Check sheet for the modelled part. Datum: model origin and axes. Units: mm. Give positions to 0.01 mm unless a question says otherwise; leave off trailing zeros. Order: outer loops, then holes, each group sorted by start corner. A loop starts at its lowest first (then second) coordinate and runs counter-clockwise, first axis right, second up. Notation, with made-up numbers: (34.5, 56.5) -> (55.5, 56.5) arc R13 ccw to (55.5, 78.5) -> close; hole circle Ø6 at (71.25, 31.25). An arc over 180 degrees is marked (long way). Answer in a Markdown table with one row per item. Add a question column.
(1) Go/stop test with flat-tipped pins: pin 1 (1.5 mm diameter, centred on x = 2, y = 5.5, fed in from -Z); pin 2 (1.5 mm diameter, centred on x = -5.5, y = 9, fed in from -Z); pin 3 (5.5 mm diameter, centred on x = 1.5, y = 5.5, fed in from -Z). Record where each tip stops, or that it passes through.
(2) Cross-section at A-A (x = -4). Record the cut outline in (y, z) (3 decimals), then the cut area to 3 significant figures.
(3) Thickness scan on L1, parallel to X at y = 8.75, z = -0.5; L2, parallel to Y at x = 4.5, z = 0.5; L3, parallel to Z at x = 1.25, y = 4.5. Record the ranges inside material, lowest first. Write a range as [from, to].
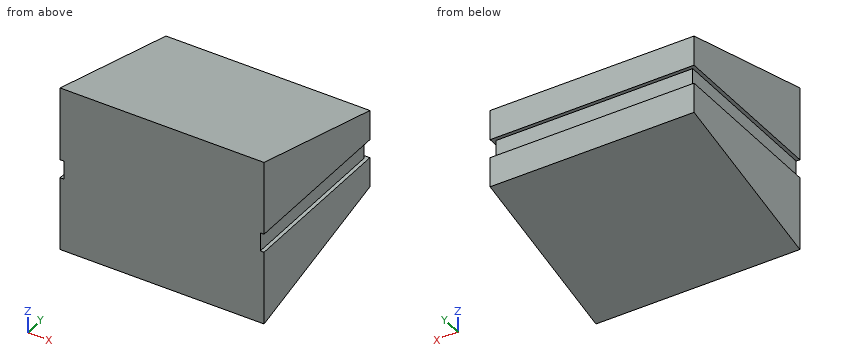
```python
from build123d import *

# Parameters (mm, degrees)
SKETCH4_W          = 13.8
SKETCH4_H          = 1.25
CUT_EXTRUDE1_DEPTH = 0.25
SKETCH5_W          = 1.25
SKETCH5_H          = 10.95
CUT_EXTRUDE2_DEPTH = 0.25
SKETCH6_W          = 1.25
SKETCH6_H          = 10.95
CUT_EXTRUDE3_DEPTH = 0.25


with BuildPart() as part:
    # Sketch1 → Loft1 section 0
    with BuildSketch(Plane(origin=(0, 0, 0), x_dir=(1, 0, 0), z_dir=(0, 1, 0))):
        with BuildLine():
            Line((-6.9, -5.61), (6.9, -5.61))
            Line((6.9, -5.61), (6.9, 5.61))
            Line((6.9, 5.61), (-6.9, 5.61))
            Line((-6.9, 5.61), (-6.9, -5.61))
        make_face()
    # Sketch2 → Loft1 section 1
    with BuildSketch(Plane(origin=(0, 11.2, 0), x_dir=(1, 0, 0), z_dir=(0, 1, 0))):
        with BuildLine():
            Line((-6.9, -2.651033308), (6.9, -2.651033308))
            Line((6.9, -2.651033308), (6.9, 2.648966692))
            Line((6.9, 2.648966692), (-6.9, 2.648966692))
            Line((-6.9, 2.648966692), (-6.9, -2.651033308))
        make_face()
    loft()

    # Sketch4 → Cut-Extrude1 (cut)
    with BuildSketch(Plane(origin=(0, 11.2, 0), x_dir=(1, 0, 0), z_dir=(0, 1, 0))):
        Rectangle(SKETCH4_W, SKETCH4_H)
    extrude(amount=-CUT_EXTRUDE1_DEPTH, mode=Mode.SUBTRACT)

    # Sketch5 → Cut-Extrude2 (cut)
    with BuildSketch(Plane(origin=(6.9, 0, 0), x_dir=(0, 0, -1), z_dir=(1, 0, 0))):
        with Locations((0, 5.475)):
            Rectangle(SKETCH5_W, SKETCH5_H)
    extrude(amount=-CUT_EXTRUDE2_DEPTH, mode=Mode.SUBTRACT)

    # Sketch6 → Cut-Extrude3 (cut)
    with BuildSketch(Plane.ZY.offset(6.9)):
        with Locations((0, 5.475)):
            Rectangle(SKETCH6_W, SKETCH6_H)
    extrude(amount=-CUT_EXTRUDE3_DEPTH, mode=Mode.SUBTRACT)


solid = part.part
```
Answer below:
| question | item | result |
|---|---|---|
| 1 | pin 1 | stops at z = -4.35 |
| 1 | pin 2 | stops at z = -3.43 |
| 1 | pin 3 | stops at z = -4.88 |
| 2 | outline | (0, -5.61) -> (11.2, -2.649) -> (11.2, -0.625) -> (10.95, -0.625) -> (10.95, 0.625) -> (11.2, 0.625) -> (11.2, 2.651) -> (0, 5.61) -> close |
| 2 | area | 92.2 mm² |
| 3 | L1 | x = [-6.65, 6.65] |
| 3 | L2 | y = [0, 10.95] |
| 3 | L3 | z = [-4.42, 4.42] |
